from build123d import *

# Parameters (mm, degrees)
BOSS_EXTRUDE1_DEPTH = 5
FILLET1_R           = 10
FILLET2_START       = -1
FILLET2_DEPTH       = 7
FILLET2_2_DEPTH     = 5
FILLET3_R           = 1
BOSS_EXTRUDE2_DEPTH = 5


with BuildPart() as part:
    # Sketch2 → Boss-Extrude1 (new body)
    with BuildSketch(Plane(origin=(0, 0, 0), x_dir=(1, 0, 0), z_dir=(0, 1, 0))):
        with BuildLine():
            add(Edge.make_bspline(
                [(-26.460947075, 51.114211153), (-12.427548014, 25.108493293), (-4.028423797, 24.103183764), (-4.41793616, 22.483556797)],
                knots=[0, 0, 0, 0, 1, 1, 1, 1], degree=3))
            add(Edge.make_bspline(
                [(-4.41793616, 22.483556797), (-4.887213543, 20.187029491), (-12.597975929, 19.976462624), (-14.992954401, 20.804801043)],
                knots=[0, 0, 0, 0, 1, 1, 1, 1], degree=3))
            add(Edge.make_bspline(
                [(-14.992954401, 20.804801043), (1.787270351, -6.103899351), (8.22123179, -2.127672237), (7.172892256, -4.601264311)],
                knots=[0, 0, 0, 0, 1, 1, 1, 1], degree=3))
            add(Edge.make_bspline(
                [(7.172892256, -4.601264311), (5.638367492, -6.681504252), (-0.799609665, -8.768183654), (-9.338641476, -7.791193384)],
                knots=[0, 0, 0, 0, 1, 1, 1, 1], degree=3))
            add(Edge.make_bspline(
                [(-9.338641476, -7.791193384), (8.962790554, -34.701758749), (15.02254586, -29.475085195), (15.060000948, -32.637388979)],
                knots=[0, 0, 0, 0, 1, 1, 1, 1], degree=3))
            add(Edge.make_bspline(
                [(-26.460947075, -45.261592135), (-9.676835521, -45.586760912), (15.687111692, -36.861745266), (15.060000948, -32.637388979)],
                knots=[0, 0, 0, 0, 1, 1, 1, 1], degree=3))
            add(Edge.make_bspline(
                [(-66.046301456, -33.30600061), (-65.977623625, -36.050325123), (-47.681674197, -45.288435387), (-26.460947075, -45.261592135)],
                knots=[0, 0, 0, 0, 1, 1, 1, 1], degree=3))
            add(Edge.make_bspline(
                [(-42.38194966, -8.050912304), (-55.265743099, -27.835283819), (-66.345571411, -30.483595462), (-66.046301456, -33.30600061)],
                knots=[0, 0, 0, 0, 1, 1, 1, 1], degree=3))
            add(Edge.make_bspline(
                [(-58.896340189, -4.69945124), (-59.030645987, -6.480678116), (-50.779962761, -9.251788646), (-42.38194966, -8.050912304)],
                knots=[0, 0, 0, 0, 1, 1, 1, 1], degree=3))
            add(Edge.make_bspline(
                [(-37.440614, 21.054048916), (-53.746480623, -7.348370101), (-58.646356675, -2.305720166), (-58.896340189, -4.69945124)],
                knots=[0, 0, 0, 0, 1, 1, 1, 1], degree=3))
            add(Edge.make_bspline(
                [(-47.800827469, 22.154310098), (-47.410404752, 20.188415441), (-42.93978555, 19.761395244), (-37.440614, 21.054048916)],
                knots=[0, 0, 0, 0, 1, 1, 1, 1], degree=3))
            add(Edge.make_bspline(
                [(-26.460947075, 51.114211153), (-43.28906286, 20.482524417), (-47.971844347, 25.301823121), (-47.800827469, 22.154310098)],
                knots=[0, 0, 0, 0, 1, 1, 1, 1], degree=3))
        make_face()
    extrude(amount=BOSS_EXTRUDE1_DEPTH)

    # Fillet1
    # the kernel refuses this fillet: 10 mm, written as the material it adds along each edge
    with BuildSketch(Plane(origin=(-26.460947075, 0, 45.261592135), x_dir=(0.9998301014874635, 0, 0.018432801186160547), z_dir=(0, 1, 0))) as fillet1_piece_1:
        with BuildLine():
            CenterArc((0.095571826, -9.99999563), FILLET1_R, 90.053566795, 1.005062424)
            ThreePointArc((-0.089183316, -0.001702498), (-0.044591398, -0.000864875), (0, 0))
            ThreePointArc((0, 0), (0.043111329, -2.0179e-05), (0.086222658, 0))
        make_face()
    extrude(amount=5)

    # Fillet2: read off the stored shape, not the designer's step
    # Fillet2 outline → Fillet2 (cut)
    with BuildSketch(Plane(origin=(0, 0, 0), x_dir=(1, 0, 0), z_dir=(0, 1, 0)).offset(FILLET2_START)):
        with BuildLine():
            add(Edge.make_bspline(
                [(-47.800827469, 22.154310098), (-47.787582934, 22.087619919), (-47.769642872, 22.022700691), (-47.747126417, 21.959559472)],
                knots=[0, 0, 0, 0, 0.033923577, 0.033923577, 0.033923577, 0.033923577], degree=3))
            ThreePointArc((-47.747126417, 21.959559472), (-47.789706131, 22.119961107), (-47.805171518, 22.285195905))
            add(Edge.make_bspline(
                [(-47.805171518, 22.285195905), (-47.80474027, 22.243126607), (-47.803285041, 22.199540953), (-47.800827469, 22.154310098)],
                knots=[0.985629653, 0.985629653, 0.985629653, 0.985629653, 1, 1, 1, 1], degree=3))
        make_face()
        with BuildLine():
            ThreePointArc((-58.480285024, -5.49409461), (-58.77681304, -4.607482629), (-58.211007375, -3.86325577))
            add(Edge.make_bspline(
                [(-58.211007375, -3.86325577), (-58.63585352, -4.060348609), (-58.849105033, -4.247148374), (-58.896340189, -4.69945124)],
                knots=[0.811046917, 0.811046917, 0.811046917, 0.811046917, 1, 1, 1, 1], degree=3))
            add(Edge.make_bspline(
                [(-58.896340189, -4.69945124), (-58.915187245, -4.949409799), (-58.768914163, -5.218861494), (-58.480285024, -5.49409461)],
                knots=[0, 0, 0, 0, 0.140329434, 0.140329434, 0.140329434, 0.140329434], degree=3))
        make_face()
        with BuildLine():
            ThreePointArc((6.603041154, -3.423142366), (7.103155792, -4.171777978), (6.798725932, -5.019063284))
            add(Edge.make_bspline(
                [(6.798725932, -5.019063284), (6.944949461, -4.880385824), (7.069953552, -4.740810579), (7.172892256, -4.601264311)],
                knots=[0.932918187, 0.932918187, 0.932918187, 0.932918187, 1, 1, 1, 1], degree=3))
            add(Edge.make_bspline(
                [(7.172892256, -4.601264311), (7.423474277, -4.01000768), (7.246561276, -3.787256085), (6.603041154, -3.423142366)],
                knots=[0, 0, 0, 0, 0.239027541, 0.239027541, 0.239027541, 0.239027541], degree=3))
        make_face()
    extrude(amount=FILLET2_DEPTH, mode=Mode.SUBTRACT)

    # Fillet2 2 outline → Fillet2 2 (add)
    with BuildSketch(Plane(origin=(0, 0, 0), x_dir=(1, 0, 0), z_dir=(0, 1, 0))):
        with BuildLine():
            add(Edge.make_bspline(
                [(-66.048164843, -33.286769384), (-66.047602355, -33.29317903), (-66.046981263, -33.299589371), (-66.046301456, -33.30600061)],
                knots=[0.997728448, 0.997728448, 0.997728448, 0.997728448, 1, 1, 1, 1], degree=3))
            ThreePointArc((-66.048164843, -33.286769384), (-66.04674894, -33.304768154), (-66.045658211, -33.322789552))
            add(Edge.make_bspline(
                [(-66.046301456, -33.30600061), (-66.046162074, -33.311570221), (-66.045947617, -33.317166579), (-66.045658211, -33.322789552)],
                knots=[0, 0, 0, 0, 0.002029502, 0.002029502, 0.002029502, 0.002029502], degree=3))
        make_face()
        with BuildLine():
            add(Edge.make_bspline(
                [(15.064825863, -32.674467974), (15.063438106, -32.662070244), (15.061830087, -32.649710467), (15.060000948, -32.637388979)],
                knots=[0.997083227, 0.997083227, 0.997083227, 0.997083227, 1, 1, 1, 1], degree=3))
            ThreePointArc((15.064825863, -32.674467974), (15.061134508, -32.634107801), (15.059081591, -32.593631201))
            add(Edge.make_bspline(
                [(15.060000948, -32.637388979), (15.059826038, -32.622621486), (15.059519797, -32.608036936), (15.059081591, -32.593631201)],
                knots=[0, 0, 0, 0, 0.004669853, 0.004669853, 0.004669853, 0.004669853], degree=3))
        make_face()
    extrude(amount=FILLET2_2_DEPTH)

    # Fillet3
    fillet3_edges = [part.edges().sort_by_distance(p)[0] for p in [
        (-26.460947075, 2.5, -51.114211153),
    ]]
    fillet(fillet3_edges, radius=FILLET3_R)

    # Sketch3 → Boss-Extrude2 (add)
    with BuildSketch(Plane(origin=(0, 5, 0), x_dir=(1, 0, 0), z_dir=(0, 1, 0))):
        Polygon((-36.595543758, -44.59706636), (-36.595543758, -58.179607966), (-16.334320806, -58.179607966), (-16.334320806, -44.578133049), align=None)
    extrude(amount=-BOSS_EXTRUDE2_DEPTH)


solid = part.part
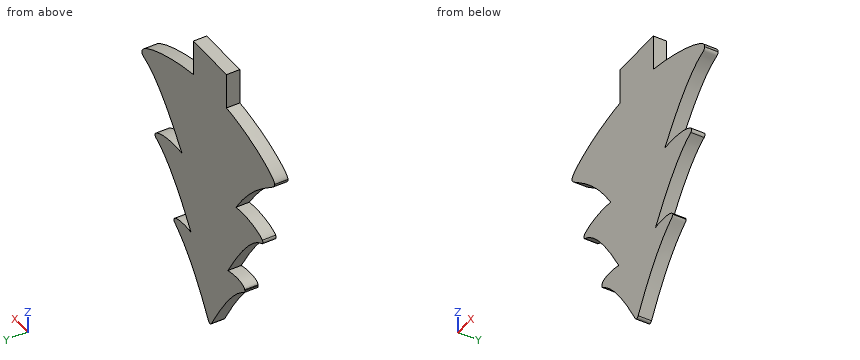
Here's how the part is built. I have some questions about the finished solid (model axes, mm). Round coordinates to 2 decimals unless told otherwise and drop trailing zeros. Order: outer loops, then holes, each group sorted by start corner. A loop starts at its lowest first (then second) coordinate and runs counter-clockwise, first axis right, second up. Notation, with made-up numbers: (58.25, -1) -> (73.25, -1) arc R20 ccw to (73.25, 23) -> close; hole circle Ø11 at (-27, 47.25). An arc over 180 degrees is marked (long way). Return JSON: item names as keys, results as strings.
Q1. I need wall thicknesses on line 1 along Z through (x, y) = (-46, 2.85); line 2 along Z through (x, y) = (-47.5, 2.35); line 3 along Z through (x, y) = (-52, 2.05). Which ranges of each line are inside material? Lowest first, please. Write a range as from..to.
Filled sheet:
{"line 1": "z = -24.31..-20.66, -7.57..8.34, 13.24..42.82", "line 2": "z = -23.21..-21.53, -5.56..8.33, 15.2..42.43", "line 3": "z = -0.37..7.88, 20.42..41.08"}
Q2. If we section it at B-B on x = -46: Give the number of separate pieces and of enclosed holes in the cut face, plus the area to 3 significant figures.
Filled sheet:
{"separate pieces": "3", "enclosed holes": "0", "area": "246 mm^2"}
Q3. If we section it at A-A on z = 51: List the corners of the cut face in (x, y) for me.
Filled sheet:
{"outline": "(-36.6, 0) -> (-16.33, 0) -> (-16.33, 5) -> (-36.6, 5) -> close"}
